Read the model definition and answer for the solid it produces. Units are mm, in the model's axes. A direction names the side the tool comes from. Round coordinates to 2 decimals unless told otherwise and drop trailing zeros. Write each loop counter-clockwise with the first axis right and the second up, starting at its lowest first coordinate (ties: lowest second). Pieces come first, ordered by that corner, then holes. Notation, with made-up numbers: (-1.5, -11.75) -> (46.5, -11.75) arc R25 ccw to (46.5, 6.25) -> close; hole circle Ø8 at (-9.75, 37.5). An arc over 180 degrees is marked (long way). Return JSON: item names as keys, results as strings.
from build123d import *
from build123d.topology import SkipClean

# Parameters (mm, degrees)
SKETCH_1_R           = 17
SKETCH_1_R_2         = 6.5
EXTRUDE_2_DEPTH      = 35
SKETCH_3_W           = 33.795275063
SKETCH_3_H           = 34.72803434
SKETCH_3_R           = 13
EXTRUDE_7_DEPTH      = 45
SKETCH_4_R           = 6.5
CUT_EXTRUDE_1_DEPTH  = 60.489495005
SKETCH_12_R          = 2
CUT_EXTRUDE_11_DEPTH = 45
SKETCH_15_R          = 2
CUT_EXTRUDE_12_DEPTH = 45
FILLET_4_R           = 10
SKETCH_20_R          = 13
CUT_EXTRUDE_18_DEPTH = 31
EXTRUDE_START        = 1
SKETCH_25_R          = 13
EXTRUDE_10_DEPTH     = 1
SKETCH_26_R          = 6.5
SKETCH_26_R_2        = 5.5
EXTRUDE_11_DEPTH     = 2


with BuildPart() as part:
    # Эскиз1 → Бобышка-Вытянуть2 (new body)
    with BuildSketch(Plane.XY):
        Circle(SKETCH_1_R)
        Circle(SKETCH_1_R_2, mode=Mode.SUBTRACT)
    extrude(amount=EXTRUDE_2_DEPTH)

    # Эскиз3 → Бобышка-Вытянуть7 (add)
    with BuildSketch(Plane(origin=(0, 45, 0), x_dir=(1, 0, 0), z_dir=(0, 1, 0))):
        with Locations((0.102362468, -17.511098906)):
            Rectangle(SKETCH_3_W, SKETCH_3_H)
        with Locations(Location((0, -17.5, 0), (0, 0, 270))):
            Circle(SKETCH_3_R, mode=Mode.SUBTRACT)
    extrude(amount=-EXTRUDE_7_DEPTH)

    # Эскиз4 → Вырез-Вытянуть1 (cut, through all)
    with BuildSketch(Plane(origin=(0, 0, 0), x_dir=(-1, 0, 0), z_dir=(0, 0, -1))):
        with Locations(Location((0, 0, 0), (0, 0, 180))):
            Circle(SKETCH_4_R)
    extrude(amount=-CUT_EXTRUDE_1_DEPTH, mode=Mode.SUBTRACT)

    # Эскиз12 → Вырез-Вытянуть11 (cut)
    with BuildSketch(Plane(origin=(0, 0, 0), x_dir=(-1, 0, 0), z_dir=(0, 0, -1))):
        with Locations((0, 23)):
            Circle(SKETCH_12_R)
    extrude(amount=-CUT_EXTRUDE_11_DEPTH, mode=Mode.SUBTRACT)

    # Эскиз15 → Вырез-Вытянуть12 (cut)
    with BuildSketch(Plane.ZY.offset(16.795275063)):
        with Locations((17.5, 33)):
            Circle(SKETCH_15_R)
    extrude(amount=-CUT_EXTRUDE_12_DEPTH, mode=Mode.SUBTRACT)

    # Скругление4
    # the kernel refuses this fillet: 10 mm, written as the material it takes off along each edge
    with BuildSketch(Plane(origin=(-16.795275063, 70, 34.875116076), x_dir=(1, 0, 0), z_dir=(0, -1, 0))) as fillet_4_piece_1_section:
        with BuildLine():
            CenterArc((FILLET_4_R, -FILLET_4_R), FILLET_4_R, 90, 90)
            Line((0, -FILLET_4_R), (0, 0))
            Line((0, 0), (FILLET_4_R, 0))
        make_face()
    fillet_4_piece_1 = extrude(amount=92.369651061, mode=Mode.PRIVATE)
    fillet_4_piece_1 = fillet_4_piece_1 - Plane(origin=(0, 0, 32.54483178), x_dir=(1, 0, 0), z_dir=(0, 0, -1)) * Cylinder(17, 225, mode=Mode.PRIVATE)
    add(fillet_4_piece_1, mode=Mode.SUBTRACT)
    with BuildSketch(Plane(origin=(17, 70, 0.147081736), x_dir=(0, 0, 1), z_dir=(0, -1, 0))) as fillet_4_piece_2_section:
        with BuildLine():
            CenterArc((FILLET_4_R, FILLET_4_R), FILLET_4_R, 180, 90)
            Line((0, FILLET_4_R), (0, 0))
            Line((0, 0), (FILLET_4_R, 0))
        make_face()
    fillet_4_piece_2 = extrude(amount=95, mode=Mode.PRIVATE)
    fillet_4_piece_2 = fillet_4_piece_2 - Plane(origin=(0, 0, 2.486350956), x_dir=(1, 0, 0), z_dir=(0, 0, -1)) * Cylinder(17, 230, mode=Mode.PRIVATE)
    add(fillet_4_piece_2, mode=Mode.SUBTRACT)
    with BuildSketch(Plane(origin=(17, 70, 34.875116076), x_dir=(0, 0, -1), z_dir=(0, -1, 0))) as fillet_4_piece_3_section:
        with BuildLine():
            CenterArc((FILLET_4_R, -FILLET_4_R), FILLET_4_R, 90, 90)
            Line((0, -FILLET_4_R), (0, 0))
            Line((0, 0), (FILLET_4_R, 0))
        make_face()
    fillet_4_piece_3 = extrude(amount=95, mode=Mode.PRIVATE)
    fillet_4_piece_3 = fillet_4_piece_3 - Plane(origin=(0, 0, 32.535846855), x_dir=(1, 0, 0), z_dir=(0, 0, -1)) * Cylinder(17, 230, mode=Mode.PRIVATE)
    add(fillet_4_piece_3, mode=Mode.SUBTRACT)
    with BuildSketch(Plane(origin=(-16.795275063, 70, 0.147081736), x_dir=(0, 0, 1), z_dir=(0, -1, 0))) as fillet_4_piece_4_section:
        with BuildLine():
            CenterArc((FILLET_4_R, -FILLET_4_R), FILLET_4_R, 90, 90)
            Line((0, -FILLET_4_R), (0, 0))
            Line((0, 0), (FILLET_4_R, 0))
        make_face()
    fillet_4_piece_4 = extrude(amount=92.369651061, mode=Mode.PRIVATE)
    fillet_4_piece_4 = fillet_4_piece_4 - Plane(origin=(0, 0, 2.477367304), x_dir=(1, 0, 0), z_dir=(0, 0, -1)) * Cylinder(17, 225, mode=Mode.PRIVATE)
    add(fillet_4_piece_4, mode=Mode.SUBTRACT)

    # Эскиз20 → Вырез-Вытянуть18 (cut)
    with SkipClean():  # the faces are left unmerged after this step: merging them gives an invalid solid
        with BuildSketch(Plane(origin=(0, 45, 0), x_dir=(1, 0, 0), z_dir=(0, 1, 0))):
            with Locations(Location((0, -17.5, 0), (0, 0, 270))):
                Circle(SKETCH_20_R)
        extrude(amount=-CUT_EXTRUDE_18_DEPTH, mode=Mode.SUBTRACT)

    # Эскиз25 → Бобышка-Вытянуть10 (add)
    with BuildSketch(Plane(origin=(0, 14, 0), x_dir=(1, 0, 0), z_dir=(0, 1, 0)).offset(EXTRUDE_START)):
        with Locations(Location((0, -17.5, 0), (0, 0, 270))):
            Circle(SKETCH_25_R)
    extrude(amount=-EXTRUDE_10_DEPTH)

    # Эскиз26 → Бобышка-Вытянуть11 (add)
    with BuildSketch(Plane(origin=(0, 0, 0), x_dir=(-1, 0, 0), z_dir=(0, 0, -1))):
        Circle(SKETCH_26_R)
        Circle(SKETCH_26_R_2, mode=Mode.SUBTRACT)
    extrude(amount=-EXTRUDE_11_DEPTH)


solid = part.part
Item 1: Section A-A (x = 0) is taken. Give the vertices of the cut face in (y, z), then the cut area to 3 significant figures.
Worked answers:
{"outline": "(-17, 0) -> (-5.5, 0) -> (-5.5, 2) -> (-6.5, 2) -> (-6.5, 35) -> (-17, 35) -> close; (5.5, 0) -> (17, 0) -> (17, 0.15) -> (21, 0.15) -> (21, 4.5) -> (15, 4.5) -> (15, 30.5) -> (21, 30.5) -> (21, 34.88) -> (17, 34.88) -> (17, 35) -> (6.5, 35) -> (6.5, 2) -> (5.5, 2) -> close; (25, 0.15) -> (45, 0.15) -> (45, 4.5) -> (25, 4.5) -> close; (25, 30.5) -> (45, 30.5) -> (45, 34.88) -> (25, 34.88) -> close", "area": "896 mm2"}
Item 2: Straight lines are drawn through the part: L1, parallel to Y at x = 0, z = 31.55; L2, parallel to Y at x = 0, z = 1; L3, parallel to Z at x = -10.5, y = 29. For each, find the intervals that lie inside material, in ascending order. Write a range as [from, to].
Worked answers:
{"L1": "y = [-17, -6.5], [6.5, 21], [25, 45]", "L2": "y = [-17, -5.5], [5.5, 21], [25, 45]", "L3": "z = [0.86, 9.84], [25.16, 34.16]"}
Item 3: Section D-D (y = 12.5) is taken. Give the vertices of the cut face in (x, z).
Worked answers:
{"outline": "(-16.8, 10.15) arc R10 ccw to (-11.52, 1.33) -> (-11.52, 0) -> (11.52, 0) -> (11.52, 1.23) arc R10 ccw to (17, 10.15) -> (17, 24.88) arc R10 ccw to (11.52, 33.79) -> (11.52, 35) -> (-11.52, 35) -> (-11.52, 33.69) arc R10 ccw to (-16.8, 24.88) -> close; hole (-11.52, 11.48) -> (-11.52, 23.52) arc R13 ccw to start; hole (11.52, 11.48) arc R13 ccw to (11.52, 23.52) -> close"}
Item 4: A tool of negligible diameter and unlimited length cuts with its end or side. For faces 4 (the cylindrical face through (11.07, 12.9, 17.38)), 5 (the cylindrical face through (-13.94, 28.82, 3.15)), 6 (the cylindrical face through (-5.158, -3.955, 18.269)), 7 (the flat face through (0, 15, 17)), 8 (the cylindrical face through (13.993, 27.815, 2.999)), from which of +Z, -Z, +X, -X, +Y, -Y can it reach the whole face along a straight path? Write none if from no direction.
Worked answers:
{"face 4": "none", "face 5": "-Z, -X, +Y", "face 6": "+Z", "face 7": "+Y", "face 8": "-Z, +X, +Y"}
Item 5: Flat-ended cylindrical pins translate along their axes: pin 1 (5 mm diameter, centred on x = -13.5, y = 3.5, fed in from -Z); pin 2 (3 mm diameter, centred on x = -13.5, z = 11, fed in from -Y); pin 3 (3 mm diameter, centred on x = -2, z = 18.5, fed in from -Y); pin 4 (1.7 mm diameter, centred on x = -11, z = 21.5, fed in from -Y). Find the tip coordinate at first contact, or state that the pin passes through.
Worked answers:
{"pin 1": "stops at z = 0", "pin 2": "stops at y = -12.04", "pin 3": "stops at y = -16.99", "pin 4": "stops at y = -13.64"}
Item 6: Section C-C (y = 27.5) is taken. Give the vertices of the cut face in (x, z).
Worked answers:
{"outline": "(-16.8, 10.15) arc R10 ccw to (-6.8, 0.15) -> (7, 0.15) arc R10 ccw to (17, 10.15) -> (17, 24.88) arc R10 ccw to (7, 34.88) -> (-6.8, 34.88) arc R10 ccw to (-16.8, 24.88) -> close; hole circle Ø26 at (0, 17.5)"}
Item 7: Section B-B (z = 17.5) is taken. Give the vertices of the cut face in (x, y).
Worked answers:
{"outline": "(-16.8, 2.63) arc R17 ccw (long way) to (17, 0) -> (17, 31) -> (13, 31) -> (13, 15) -> (-13, 15) -> (-13, 31) -> (-16.8, 31) -> close; (-16.8, 35) -> (-13, 35) -> (-13, 45) -> (-16.8, 45) -> close; (13, 35) -> (17, 35) -> (17, 45) -> (13, 45) -> close; hole (-13, 10.95) arc R17 cw to (-9.64, 14) -> (-13, 14) -> close; hole circle Ø13 at (0, 0); hole (9.64, 14) arc R17 cw to (13, 10.95) -> (13, 14) -> close"}
Item 8: For a pull along X with two mould halves and no side action, classify faces 1 (the flat face through (-11, 14, 17)), 2 (the flat face through (7, 0, 35)), 3 (the cylindrical face through (14.148, 27.815, 31.868)) as released by +X, released by -X, zero draft, split by the parting line, or undercut.
Worked answers:
{"face 1": "undercut", "face 2": "zero draft", "face 3": "released by +X"}
